Could you check a few things on this model? Use its own coordinates, in mm. Give positions to 0.01 mm unless a question says otherwise; leave off trailing zeros. Loops run counter-clockwise (first coordinate to the right, second up) from the corner with the lowest first, then second, coordinate; pieces in that order, holes last. Notation, with made-up numbers: (89.25, 3) - (129.25, 3) arc R16 cw to (129.25, 7) - close; hole circle Ø7 at (23, 30.5). An arc over 180 degrees is marked (long way). Write each question's results on one line, items separated by ' | '. Start each with the question number.
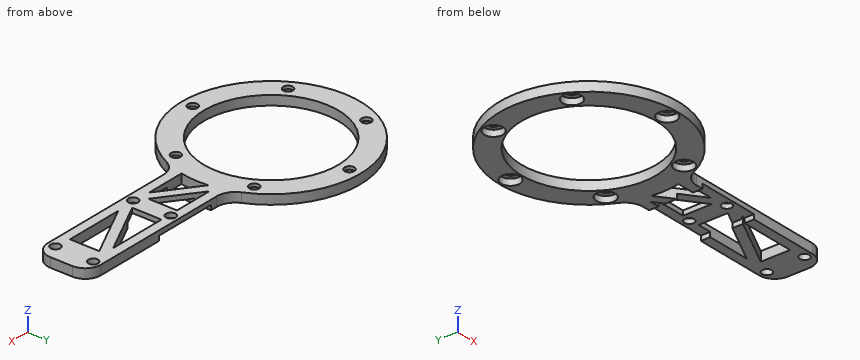
Autodesk Inventor part; units mm, degrees
ref_plane "YZ Plane" through (0, 0, 0) normal (1, 0, 0) x (0, 1, 0)
ref_plane "XZ Plane" through (0, 0, 0) normal (0, 1, 0) x (-1, 0, 0)
ref_plane "XY Plane" through (0, 0, 0) normal (0, 0, 1) x (1, 0, 0)
sketch "スケッチ1" plane through (0, 0, 0) normal (0, 0, 1) x (1, 0, 0)
  line L0 (0, 0) -> (-109.5, 0)
  line L1 (-109.5, 0) -> (-109.5, 17)
  line L2 (-109.5, 17) -> (0, 17)
  line L3 (0, 17) -> (0, 0)
  line L4 (0, 8.5) -> (-109.5, 8.5)
  circle A0 centre (-81, 8.5) radius 28.5
  point P0 (-53.7971, 17)
  point P1 (-53.7971, 0)
  dimension "d0" = 17
  dimension "d48" = 57
  dimension "d51" = 81
extrude "押し出し1" add sketch "スケッチ1" along normal blind 3 contours L0 A0 L4 L3 | A0 L0 | L0 A0 L4 | L4 A0 L2 L3 | L4 A0 L2 | L2 A0
sketch "スケッチ2" plane through (0, 0, 3) normal (0, 0, 1) x (1, 0, 0)
  line L0 (0, 17) -> (-53.7971, 17)
  line L1 (-5, 17) -> (-5, 0)
  line L2 (-53.7971, 0) -> (0, 0)
  line L3 (-35, 17) -> (-35, 0)
  line L4 (0, 0) -> (0, 17)
  line L5 (0, 8.5) -> (-5, 8.5)
  line L6 (-35, 17) -> (-53.7971, 17)
  point P0 (-5, 14.5)
  point P1 (-35, 14.5)
  point P2 (-5, 2.5)
  point P3 (-35, 2.5)
  dimension "d4" = 5
  dimension "d5" = 30
  dimension "d49" = 6
  dimension "d50" = 6
hole "穴1" at (-5, 14.5, 3) at (-35, 14.5, 3) at (-5, 2.5, 3) at (-35, 2.5, 3) direction (0, 0, -1) diameter 3.1 depth 20 tip angle 118
sketch "スケッチ7" plane through (0, 0, 0) normal (0, 0, -1) x (-1, 0, 0)
  arc A0 (53.7971, 0) -> (53.7971, 17) centre (81, 8.5) ccw
  circle A1 centre (81, 8.5) radius 25
  line L0 (81, 8.5) -> (81, 33.5)
  line L1 (81, 8.5) -> (81, 33.5)
  point P0 (0, 0)
  point P1 (81, 33.5)
  point P2 (59.3494, 21)
  point P3 (59.3494, -4)
  point P4 (81, -16.5)
  point P5 (102.6506, -4)
  point P6 (102.6506, 21)
  dimension "d52" = 50
  dimension "d55" = 360
  dimension "d75" = 0
hole "穴3" at (-81, 33.5, 0) at (-59.3494, 21, 0) at (-59.3494, -4, 0) at (-81, -16.5, 0) at (-102.6506, -4, 0) at (-102.6506, 21, 0) direction (0, 0, 1) diameter 3.1 end through all
sketch "スケッチ8" plane through (0, 0, 0) normal (0, 0, -1) x (-1, 0, 0)
  arc A0 (53.7971, 0) -> (53.7971, 17) centre (81, 8.5) ccw
  circle A1 centre (81, 8.5) radius 21.5
  point P0 (0, 0)
  dimension "d64" = 43
extrude "押し出し5" cut sketch "スケッチ8" against normal blind 3
sketch "スケッチ9" plane through (0, 0, 0) normal (0, 0, -1) x (-1, 0, 0)
  circle A0 centre (59.3494, -4) radius 1.55
  circle A1 centre (59.3494, -4) radius 3
  circle A2 centre (59.3494, 21) radius 1.55
  circle A3 centre (59.3494, 21) radius 3
  circle A4 centre (81, 33.5) radius 1.55
  circle A5 centre (81, 33.5) radius 3
  circle A6 centre (102.6506, 21) radius 1.55
  circle A7 centre (102.6506, 21) radius 3
  circle A8 centre (102.6506, -4) radius 1.55
  circle A9 centre (102.6506, -4) radius 3
  circle A10 centre (81, -16.5) radius 1.55
  circle A11 centre (81, -16.5) radius 3
  point P0 (0, 0)
  dimension "d67" = 6
  dimension "d68" = 6
  dimension "d69" = 6
  dimension "d70" = 6
  dimension "d71" = 6
  dimension "d72" = 6
extrude "押し出し6" cut sketch "スケッチ9" against normal blind 2 contours A1 | A2 | A3 | A4 | A5 | A6 | A7 | A8 | A9 | A10 | A11
sketch "スケッチ10" plane through (0, 0, 0) normal (0, 0, -1) x (-1, 0, 0)
  line L0 (0, 17) -> (53.7971, 17)
  line L1 (10, 17) -> (10, 0)
  line L2 (0, 0) -> (0, 17)
  line L3 (53.7971, 0) -> (0, 0)
  line L4 (32, 17) -> (38, 17)
  line L5 (38, 17) -> (38, 0)
  line L6 (38, 0) -> (32, 0)
  line L7 (32, 0) -> (32, 17)
  line L8 (10, 3) -> (53.0357, 3)
  line L9 (10, 14) -> (38, 14)
  arc A0 (53.7971, 0) -> (53.7971, 17) centre (81, 8.5) ccw
  circle A1 centre (81, 8.5) radius 28.5
  line L10 (38, 14) -> (53.0357, 14)
  line L11 (53.0357, 14) -> (38, 3)
  line L12 (50.4953, 14) -> (38, 4.8586)
  line L13 (40.5404, 3) -> (52.7033, 11.8982)
  line L14 (10, 14) -> (32, 3)
  line L15 (13.3541, 14) -> (32, 4.6771)
  line L16 (10, 12.3229) -> (28.6459, 3)
  point P0 (35, 6.5)
  point P1 (32, 14)
  dimension "d76" = 10
  dimension "d77" = 3
  dimension "d78" = 3
  dimension "d79" = 3
  dimension "d80" = 3
  dimension "d81" = 1.5
  dimension "d82" = 1.5
  dimension "d83" = 1.5
  dimension "d84" = 1.5
extrude "押し出し7" cut sketch "スケッチ10" against normal blind 3 contours L7 L15 L9 | L16 L8 L1 | L10 L12 L5 | L13 A1 L8
fillet "フィレット1" radius 6 2 edges at (-53.7971, 0, 1.5) (-53.7971, 17, 1.5)
fillet "フィレット2" radius 5 2 edges at (0, 17, 1.5) (0, 0, 1.5)
sketch "スケッチ11" plane through (0, 0, 0) normal (0, 0, -1) x (-1, 0, 0)
  line L0 (5, 17) -> (49.695, 17)
  line L1 (27.5, 17) -> (47.5, 17)
  line L2 (47.5, 17) -> (47.5, 0)
  line L3 (47.5, 0) -> (27.5, 0)
  line L4 (27.5, 0) -> (27.5, 17)
  line L5 (0, 5) -> (0, 12)
  line L6 (47.5, 17) -> (47.5, 17.4159)
  arc A0 (49.695, 17) -> (55.1394, 20.4783) centre (49.695, 23) ccw
  line L7 (47.5, 0) -> (47.5, -0.4159)
  arc A1 (55.1394, -3.4783) -> (49.695, 0) centre (49.695, -6) ccw
  point P0 (0, 0)
  point P1 (47.5, 17)
  point P2 (46.695, 17)
  dimension "d89" = 27.5
  dimension "d90" = 20
extrude "押し出し8" cut sketch "スケッチ11" against normal blind 1.5
properties part number "link2plate3" material "アルミニウム 6061"
Q1. I'm going to push flat-ended pins straight in: pin 1 Ø1 at (x, z) = (-70.5, 0.5) entering from +Y; pin 2 Ø0.9 at (x, z) = (-44, 2) entering from -Y; pin 3 Ø2.5 at (x, y) = (-102.65, -4) entering from +Z; pin 4 Ø1.8 at (x, y) = (-82.5, 33.5) entering from -Z. Where does each tip first touch, or does it pass through?
Q2. I need wall thicknesses on L1, parallel to Y at x = -81, z = 2.55; L2, parallel to X at y = 6.5, z = 2.2; L3, parallel to Y at x = -81.5, z = 0.9. Which ranges of each line are inside material? Lowest first, please. Write a range as from..to.
Q3. I want a section at A-A, the plane x = -81. List the corners of the cut face in (y, z) for me.
Q4. I want a section at C-C, the plane x = -18. List the corners of the cut face in (y, z) for me, then the cut area to 3 significant figures.
Q5. I want a section at B-B, the plane x = -66.5. List the corners of the cut face in (y, z) for me.
Conclusion:
1) pin 1: y = 35.19 | pin 2: y = 0 | pin 3: through | pin 4: z = 2
2) L1: -20..-18.05, -14.95..-13, 30..31.95, 35.05..37 | L2: -109.43..-102.41, -59.59..-52.57, -45.32..-40.24, -38..-32, -28.35..-21.65, -10..0 | L3: -20..-19.46, -13.54..-12.99, 29.99..30.54, 36.46..37
3) outline: (-20, 0) - (-19.5, 0) - (-19.5, 2) - (-18.05, 2) - (-18.05, 3) - (-20, 3) - close; (-14.95, 2) - (-13.5, 2) - (-13.5, 0) - (-13, 0) - (-13, 3) - (-14.95, 3) - close; (30, 0) - (30.5, 0) - (30.5, 2) - (31.95, 2) - (31.95, 3) - (30, 3) - close; (35.05, 2) - (36.5, 2) - (36.5, 0) - (37, 0) - (37, 3) - (35.05, 3) - close
4) outline: (0, 0) - (3, 0) - (3, 3) - (0, 3) - close; (8.32, 0) - (11.68, 0) - (11.68, 3) - (8.32, 3) - close; (14, 0) - (17, 0) - (17, 3) - (14, 3) - close | area: 28.1 mm^2
5) outline: (-16.04, 0) - (-7.37, 0) - (-7.37, 3) - (-16.04, 3) - close; (24.37, 0) - (33.04, 0) - (33.04, 3) - (24.37, 3) - close
